```python
from build123d import *

# Parameters (mm, degrees)
SKETCH1_W               = 20.32
SKETCH1_H               = 10.668
BASE_DEPTH              = 5.08
BOXSLOTS_DEPTH          = 2.286
MOUTINGHOLE_D           = 3.6576
MOUTINGHOLE_CBORE_D     = 7.14502
MOUTINGHOLE_CBORE_DEPTH = 2.54
CUT_EXTRUDE1_DEPTH      = 2.286


with BuildPart() as part:
    # Sketch1 → Base (new body)
    with BuildSketch(Plane(origin=(0, 0, 0), x_dir=(1, 0, 0), z_dir=(0, 1, 0))):
        Rectangle(SKETCH1_W, SKETCH1_H)
    extrude(amount=BASE_DEPTH)

    # Sketch2 → BoxSlots (cut)
    with BuildSketch(Plane.XZ):
        with BuildLine():
            Line((-4.937125, 5.334), (-4.937125, 3.8608))
            ThreePointArc((-4.937125, 3.8608), (-5.334, 3.463925), (-5.730875, 3.8608))
            Line((-5.730875, 3.8608), (-5.730875, 5.334))
            ThreePointArc((-5.730875, 5.334), (-5.334, 5.730875), (-4.937125, 5.334))
        make_face()
        with BuildLine():
            Line((5.730875, 5.334), (5.730875, 3.8608))
            ThreePointArc((5.730875, 3.8608), (5.334, 3.463925), (4.937125, 3.8608))
            Line((4.937125, 3.8608), (4.937125, 5.334))
            ThreePointArc((4.937125, 5.334), (5.334, 5.730875), (5.730875, 5.334))
        make_face()
    extrude(amount=-BOXSLOTS_DEPTH, mode=Mode.SUBTRACT)

    # MoutingHole (through all)
    with Locations(Plane(origin=(0, 5.08, 0), x_dir=(1, 0, 0), z_dir=(0, 1, 0))):
        with Locations((0, 0)):
            CounterBoreHole(MOUTINGHOLE_D / 2, MOUTINGHOLE_CBORE_D / 2, MOUTINGHOLE_CBORE_DEPTH)

    # Sketch7 → Cut-Extrude1 (cut)
    with BuildSketch(Plane.XZ):
        with BuildLine():
            Line((-3.175, 5.334), (3.175, 5.334))
            Line((3.175, 5.334), (3.175, 4.3815))
            ThreePointArc((3.175, 4.3815), (2.710032015, 3.258967985), (1.5875, 2.794))
            Line((1.5875, 2.794), (-1.5875, 2.794))
            ThreePointArc((-1.5875, 2.794), (-2.710032015, 3.258967985), (-3.175, 4.3815))
            Line((-3.175, 4.3815), (-3.175, 5.334))
        make_face()
    extrude(amount=-CUT_EXTRUDE1_DEPTH, mode=Mode.SUBTRACT)


solid = part.part
```
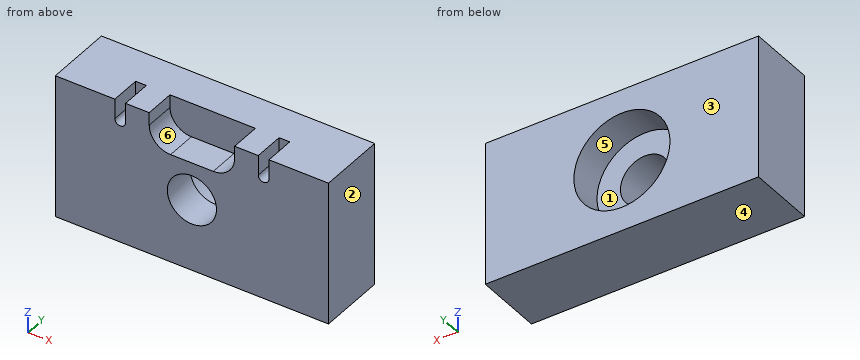
The listing builds one solid part. Answer for the finished solid, in the listing's coordinates (mm). Face numbers are marked on the shaded views. A direction names the side the tool comes from. Give positions to 0.01 mm unless a question says otherwise; leave off trailing zeros. Loops run counter-clockwise (first coordinate to the right, second up) from the corner with the lowest first, then second, coordinate; pieces in that order, holes last. Notation, with made-up numbers: (49, -14.5) - (79, -14.5) arc R31 ccw to (79, 22.5) - close; hole circle Ø6 at (-7, 8.25). An arc over 180 degrees is marked (long way). Answer as CSV lines item,"result". Start each with the question number.
Item 1: For the marked faces 4, 5 and 6, determine the directions among +Z, -Z, +X, -X, +Y, -Y from which every point of the face is accessible in a straight line to the end or side of a thin tool.
Item 2: A cutting plane is placed at C-C on y = 0.35. Determine the outline of the cut face in (x, z) (1 decimal), then the cut area to 3 significant figures.
Item 3: Find the intervals of material crossed by line 1 (Z direction, x = 0, y = 4.55); line 2 (Z direction, x = 0, y = 0.6); line 3 (Y direction, x = 2, z = 2.5), in increasing order. Write a range as from..to.
Item 4: A cutting plane is placed at D-D on z = -3. Determine the outline of the cut face in (x, y).
Item 5: The mould has two halves that part along X. Classify the marked faces 1, 2 and 3: +X half, -X half, draft (parallel to the pull), parting line (faces both ways), or undercut.
Item 6: A cutting plane is placed at B-B on x = 0. Determine the outline of the cut face in (y, z).
Item 7: A cutting plane is placed at A-A on z = 0. Determine the outline of the cut face in (x, y).
Item 8: This flat-tipped pin is pushed along its axis until it touches: pin 1 (0.8 mm diameter, centred on x = 1.5, z = 3.5, fed in from -Y). Where does it stop, or does it pass through?
Found:
1,face 4,"-Z, +X, -X, +Y, -Y"
1,face 5,"+Y"
1,face 6,"+Z, -Y"
2,outline,"(-10.2, -5.3) - (10.2, -5.3) - (10.2, 5.3) - (5.7, 5.3) - (5.7, 3.9) arc R0.4 cw to (4.9, 3.9) - (4.9, 5.3) - (3.2, 5.3) - (3.2, 4.4) arc R1.6 cw to (1.6, 2.8) - (-1.6, 2.8) arc R1.6 cw to (-3.2, 4.4) - (-3.2, 5.3) - (-4.9, 5.3) - (-4.9, 3.9) arc R0.4 cw to (-5.7, 3.9) - (-5.7, 5.3) - (-10.2, 5.3) - close; hole circle Ø3.7 at (0, 0)"
2,area,"188 mm^2"
3,line 1,"z = -5.33..-3.57, 3.57..5.33"
3,line 2,"z = -5.33..-1.83, 1.83..2.79"
3,line 3,"y = 0..2.54"
4,outline,"(-10.16, 0) - (10.16, 0) - (10.16, 5.08) - (1.94, 5.08) - (1.94, 2.54) - (-1.94, 2.54) - (-1.94, 5.08) - (-10.16, 5.08) - close"
5,face 1,"undercut"
5,face 2,"+X half"
5,face 3,"draft"
6,outline,"(0, -5.33) - (5.08, -5.33) - (5.08, -3.57) - (2.54, -3.57) - (2.54, -1.83) - (0, -1.83) - close; (0, 1.83) - (2.54, 1.83) - (2.54, 3.57) - (5.08, 3.57) - (5.08, 5.33) - (2.29, 5.33) - (2.29, 2.79) - (0, 2.79) - close"
7,outline,"(-10.16, 0) - (-1.83, 0) - (-1.83, 2.54) - (-3.57, 2.54) - (-3.57, 5.08) - (-10.16, 5.08) - close; (1.83, 0) - (10.16, 0) - (10.16, 5.08) - (3.57, 5.08) - (3.57, 2.54) - (1.83, 2.54) - close"
8,pin 1,"stops at y = 2.29"
